For this review, take the finished solid that the model builds, in its own axes (mm). Face numbers are marked on the shaded views. A direction names the side the tool comes from. Give positions to 0.01 mm unless a question says otherwise; leave off trailing zeros. Loops run counter-clockwise (first coordinate to the right, second up) from the corner with the lowest first, then second, coordinate; pieces in that order, holes last.
```python
from build123d import *

# Parameters (mm, degrees)
F1_DEPTH  = 25.4
F2_R      = 3.81
F3_DEPTH  = 12.7
F4_R      = 3.81
F5_DEPTH  = 12.7
F6_R      = 3.81
F7_DEPTH  = 12.7
F8_R      = 3.81
F9_DEPTH  = 12.7
F10_R     = 3.81
F11_DEPTH = 12.7
F12_R     = 3.81
F13_DEPTH = 12.7
F14_R     = 3.81
F15_DEPTH = 12.7
F16_R     = 3.81
F17_DEPTH = 12.7
F18_R     = 3.81
F19_DEPTH = 12.7
F20_R     = 3.81
F21_DEPTH = 12.7
F22_R     = 3.81
F23_DEPTH = 12.7
F24_R     = 3.81
F25_DEPTH = 7.62
F26_R     = 3.81
F27_DEPTH = 12.7
F28_R     = 3.81
F29_DEPTH = 12.7
F30_R     = 3.81
F31_DEPTH = 12.7
F33_DEPTH = 127


with BuildPart() as f1:
    # F0 (on Front) → F1 (new body)
    with BuildSketch(Plane.XZ):
        Polygon((-76.988041, 0), (0, 0), (-39.573293, 76.124623), align=None)
    extrude(amount=F1_DEPTH)

    # F2 (on face) → F3 (cut)
    with BuildSketch(Plane.XZ.offset(25.4)):
        with Locations((-39.679505, 60.870919)):
            Circle(F2_R)
    extrude(amount=-F3_DEPTH, mode=Mode.SUBTRACT)

    # F4 (on face) → F5 (cut)
    with BuildSketch(Plane.XZ.offset(25.4)):
        with Locations((-46.011232, 47.919661)):
            Circle(F4_R)
    extrude(amount=-F5_DEPTH, mode=Mode.SUBTRACT)

    # F6 (on face) → F7 (cut)
    with BuildSketch(Plane.XZ.offset(25.4)):
        with Locations((-33.347782, 47.919661)):
            Circle(F6_R)
    extrude(amount=-F7_DEPTH, mode=Mode.SUBTRACT)

    # F8 (on face) → F9 (cut)
    with BuildSketch(Plane.XZ.offset(25.4)):
        with Locations((-52.342959, 36.40743)):
            Circle(F8_R)
    extrude(amount=-F9_DEPTH, mode=Mode.SUBTRACT)

    # F10 (on face) → F11 (cut)
    with BuildSketch(Plane.XZ.offset(25.4)):
        with Locations((-39.679505, 36.695234)):
            Circle(F10_R)
    extrude(amount=-F11_DEPTH, mode=Mode.SUBTRACT)

    # F12 (on face) → F13 (cut)
    with BuildSketch(Plane.XZ.offset(25.4)):
        with Locations((-27.016053, 37.270848)):
            Circle(F12_R)
    extrude(amount=-F13_DEPTH, mode=Mode.SUBTRACT)

    # F14 (on face) → F15 (cut)
    with BuildSketch(Plane.XZ.offset(25.4)):
        with Locations((-57.523463, 26.334228)):
            Circle(F14_R)
    extrude(amount=-F15_DEPTH, mode=Mode.SUBTRACT)

    # F16 (on face) → F17 (cut)
    with BuildSketch(Plane.XZ.offset(25.4)):
        with Locations((-45.723427, 26.909837)):
            Circle(F16_R)
    extrude(amount=-F17_DEPTH, mode=Mode.SUBTRACT)

    # F18 (on face) → F19 (cut)
    with BuildSketch(Plane.XZ.offset(25.4)):
        with Locations((-33.059973, 26.909837)):
            Circle(F18_R)
    extrude(amount=-F19_DEPTH, mode=Mode.SUBTRACT)

    # F20 (on face) → F21 (cut)
    with BuildSketch(Plane.XZ.offset(25.4)):
        with Locations((-21.259937, 27.197644)):
            Circle(F20_R)
    extrude(amount=-F21_DEPTH, mode=Mode.SUBTRACT)

    # F22 (on face) → F23 (cut)
    with BuildSketch(Plane.XZ.offset(25.4)):
        with Locations((-61.552744, 16.261026)):
            Circle(F22_R)
    extrude(amount=-F23_DEPTH, mode=Mode.SUBTRACT)

    # F24 (on face) → F25 (cut)
    with BuildSketch(Plane.XZ.offset(25.4)):
        with Locations((-51.191736, 16.548831)):
            Circle(F24_R)
    extrude(amount=-F25_DEPTH, mode=Mode.SUBTRACT)

    # F26 (on face) → F27 (cut)
    with BuildSketch(Plane.XZ.offset(25.4)):
        with Locations((-38.528282, 16.548831)):
            Circle(F26_R)
    extrude(amount=-F27_DEPTH, mode=Mode.SUBTRACT)

    # F28 (on face) → F29 (cut)
    with BuildSketch(Plane.XZ.offset(25.4)):
        with Locations((-26.728246, 17.412249)):
            Circle(F28_R)
    extrude(amount=-F29_DEPTH, mode=Mode.SUBTRACT)

    # F30 (on face) → F31 (cut)
    with BuildSketch(Plane.XZ.offset(25.4)):
        with Locations((-16.367238, 17.124442)):
            Circle(F30_R)
    extrude(amount=-F31_DEPTH, mode=Mode.SUBTRACT)

    # F32 (on face) → F33 (cut)
    with BuildSketch(Plane.XZ.offset(25.4)):
        Polygon((-5.083223, 9.778273), (-72.182085, 9.778273), (-76.988041, 0), (0, 0), align=None)
    extrude(amount=-F33_DEPTH, mode=Mode.SUBTRACT)


solid = f1.part
```
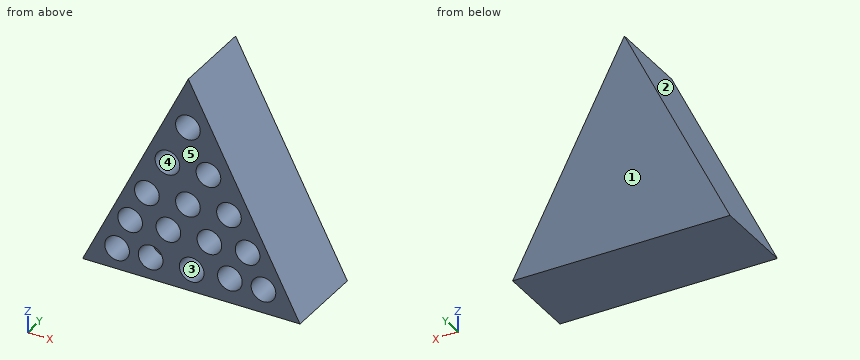
Q1. Machinability: for the marked faces 4 and 5, which of the approach directions +Z, -Z, +X, -X, +Y, -Y give a long, thin tool a straight path to every point of the face, cutting with its end or side? Answer none if there is none.
Answers:
face 4: -Y
face 5: +Z, -Z, +X, -X, -Y
Q2. Consider section B-B on z = 25. Give the boundary of the cut face in (x, y), plus the area to 3 significant figures.
Answers:
outline: (-64.7, -25.4) - (-61.09, -25.4) - (-61.09, -12.7) - (-53.95, -12.7) - (-53.95, -25.4) - (-49.02, -25.4) - (-49.02, -12.7) - (-42.43, -12.7) - (-42.43, -25.4) - (-36.36, -25.4) - (-36.36, -12.7) - (-29.76, -12.7) - (-29.76, -25.4) - (-24.37, -25.4) - (-24.37, -12.7) - (-18.15, -12.7) - (-18.15, -25.4) - (-13, -25.4) - (-13, 0) - (-64.7, 0) - close
area: 976 mm2
Q3. For pin 1 Ø5 at (x, y) = (-19, -8) entering from +Z; pin 2 Ø4 at (x, z) = (-17.5, 15.5) entering from -Y; pin 3 Ø4 at (x, y) = (-54.5, -12) entering from +Z; pin 4 Ø1 at (x, y) = (-56, -5) entering from +Z, all flat-tipped, find the tip position at first contact; note any pin that passes through.
Answers:
pin 1: stops at z = 41.36
pin 2: stops at y = -25.4
pin 3: stops at z = 49.82
pin 4: stops at z = 43.72
Q4. For probe 1 along Z at (x, y) = (-34, -19.25); probe 2 along Y at (x, z) = (-31.5, 27); probe 3 along Z at (x, y) = (-60, -15.25), list the stretches that pass through material, from the lowest coordinate up.
Answers:
probe 1: z = 9.78 to 23.22, 30.6 to 44.17, 51.67 to 65.4
probe 2: y = -12.7 to 0
probe 3: z = 9.78 to 12.78, 19.74 to 23.44, 29.23 to 34.56
Q5. Consider section A-A on x = -59. Give the boundary of the cut face in (y, z).
Answers:
outline: (-25.4, 9.78) - (0, 9.78) - (0, 36.6) - (-25.4, 36.6) - (-25.4, 29.85) - (-12.7, 29.85) - (-12.7, 22.82) - (-25.4, 22.82) - (-25.4, 19.09) - (-12.7, 19.09) - (-12.7, 13.43) - (-25.4, 13.43) - close
Q6. Mouldability with a two-part tool opening along Z and no side actions: class the marked faces 1, 2 and 3 as +Z half, -Z half, draft (parallel to the pull), parting line (faces both ways), or undercut.
Answers:
face 1: draft
face 2: +Z half
face 3: undercut
Q7. Consider section C-C on y = -16.5. Count the separate pieces of the cut face and the enclosed holes in it, plus the area to 3 significant figures.
Answers:
separate pieces: 1
enclosed holes: 14
area: 1,590 mm2
